from build123d import *

# Parameters (mm, degrees)
IZIM1_W               = 34
IZIM1_H               = 54
IZIM1_W_2             = 30
IZIM1_H_2             = 50
EKSTR_ZYON_NCE1_DEPTH = 50
KES_EKSTR_ZYON1_REACH = 81.75
IZIM2_R               = 4
IZIM2_R_2             = 2
EKSTR_ZYON_NCE2_DEPTH = 27


with BuildPart() as part:
    # Çizim1 → Ekstrüzyon-İnce1 (new body)
    with BuildSketch(Plane.XY):
        with Locations((15, 25)):
            Rectangle(IZIM1_W, IZIM1_H)
        with Locations((15, 25)):
            Rectangle(IZIM1_W_2, IZIM1_H_2, mode=Mode.SUBTRACT)
    extrude(amount=EKSTR_ZYON_NCE1_DEPTH)

    # Çizim2 → Kes-Ekstrüzyon1 (cut, up to next)
    with BuildSketch(Plane.ZY.offset(2), mode=Mode.PRIVATE) as kes_ekstr_zyon1_sk1:
        with Locations((25, 25)):
            Circle(IZIM2_R)
    kes_ekstr_zyon1_tool1 = extrude(kes_ekstr_zyon1_sk1.sketch, amount=-KES_EKSTR_ZYON1_REACH, mode=Mode.PRIVATE) & part.part
    # Çizim2 → Kes-Ekstrüzyon1 (cut, up to next)
    with BuildSketch(Plane.ZY.offset(2), mode=Mode.PRIVATE) as kes_ekstr_zyon1_sk2:
        with Locations((33, 25)):
            Circle(IZIM2_R_2)
    kes_ekstr_zyon1_tool2 = extrude(kes_ekstr_zyon1_sk2.sketch, amount=-KES_EKSTR_ZYON1_REACH, mode=Mode.PRIVATE) & part.part
    # Çizim2 → Kes-Ekstrüzyon1 (cut, up to next)
    with BuildSketch(Plane.ZY.offset(2), mode=Mode.PRIVATE) as kes_ekstr_zyon1_sk3:
        with Locations(Location((17, 25, 0), (0, 0, 180))):
            Circle(IZIM2_R_2)
    kes_ekstr_zyon1_tool3 = extrude(kes_ekstr_zyon1_sk3.sketch, amount=-KES_EKSTR_ZYON1_REACH, mode=Mode.PRIVATE) & part.part
    # Çizim2 → Kes-Ekstrüzyon1 (cut, up to next)
    with BuildSketch(Plane.ZY.offset(2), mode=Mode.PRIVATE) as kes_ekstr_zyon1_sk4:
        with Locations((25, 33)):
            Circle(IZIM2_R_2)
    kes_ekstr_zyon1_tool4 = extrude(kes_ekstr_zyon1_sk4.sketch, amount=-KES_EKSTR_ZYON1_REACH, mode=Mode.PRIVATE) & part.part
    # Çizim2 → Kes-Ekstrüzyon1 (cut, up to next)
    with BuildSketch(Plane.ZY.offset(2), mode=Mode.PRIVATE) as kes_ekstr_zyon1_sk5:
        with Locations(Location((25, 17, 0), (0, 0, 180))):
            Circle(IZIM2_R_2)
    kes_ekstr_zyon1_tool5 = extrude(kes_ekstr_zyon1_sk5.sketch, amount=-KES_EKSTR_ZYON1_REACH, mode=Mode.PRIVATE) & part.part
    add(kes_ekstr_zyon1_tool1.solids().sort_by_distance((-2, 25, 25))[0], mode=Mode.SUBTRACT)
    add(kes_ekstr_zyon1_tool2.solids().sort_by_distance((-2, 25, 33))[0], mode=Mode.SUBTRACT)
    add(kes_ekstr_zyon1_tool3.solids().sort_by_distance((-2, 25, 17))[0], mode=Mode.SUBTRACT)
    add(kes_ekstr_zyon1_tool4.solids().sort_by_distance((-2, 33, 25))[0], mode=Mode.SUBTRACT)
    add(kes_ekstr_zyon1_tool5.solids().sort_by_distance((-2, 17, 25))[0], mode=Mode.SUBTRACT)

    # Çizim3 → Ekstrüzyon-İnce2 (add, symmetric)
    with BuildSketch(Plane(origin=(0, 52, 0), x_dir=(1, 0, 0), z_dir=(0, 1, 0))):
        with BuildLine():
            ThreePointArc((25.118164338, -77.900907107), (30.254140884, -64.368544459), (32, -50))
            Line((32, -50), (32, 0))
            ThreePointArc((32, 0), (30.254140884, 14.368544459), (25.118164338, 27.900907107))
            Line((25.118164338, 27.900907107), (27.774072555, 29.295952462))
            ThreePointArc((27.774072555, 29.295952462), (33.166847928, 15.086971682), (35, 0))
            Line((35, 0), (35, -50))
            ThreePointArc((35, -50), (33.166847928, -65.086971682), (27.774072555, -79.295952462))
            Line((27.774072555, -79.295952462), (25.118164338, -77.900907107))
        make_face()
    ekstr_zyon_nce2 = extrude(amount=EKSTR_ZYON_NCE2_DEPTH, both=True)

    # Aynalama1: Ekstrüzyon-İnce2 across plane
    add(ekstr_zyon_nce2.mirror(Plane(origin=(-28, 25, 50), x_dir=(0, 0, 1), z_dir=(0, -1, 0))))


solid = part.part
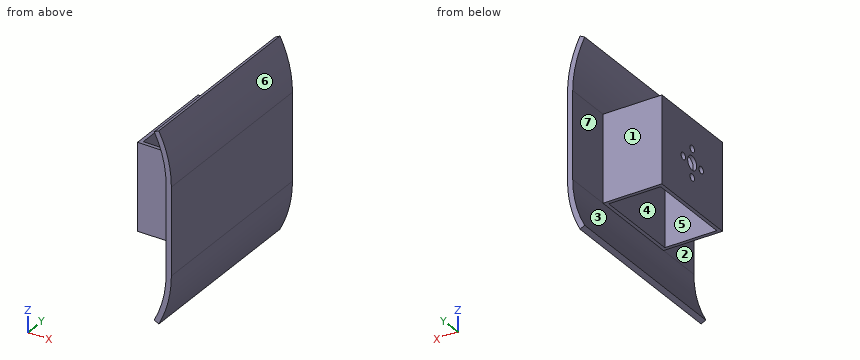
Here's how the part is built. I have some questions about the finished solid (model axes, mm). Face numbers are marked on the shaded views. A direction names the side the tool comes from. Coordinates: 2 decimals unless noted, no trailing zeros. Loops run counter-clockwise (first coordinate to the right, second up) from the corner with the lowest first, then second, coordinate; pieces in that order, holes last.
1. I need wall thicknesses on L1, parallel to X at y = 47, z = 38; L2, parallel to Y at x = 15.5, z = 16.5; L3, parallel to Z at x = -0.9, y = 17. Which ranges of each line are inside material? Lowest first, please.
2. Imagine slicing it at C-C, the plane z = 25. Please give me the cut outline in (x, y), and give its area (3 significant figures).
3. For P1, Ø10, axis at y = 58.5, z = -5.5, coming from the +X side; P2, Ø8, axis at y = 7, z = 64.5, coming from the -X side; P3, Ø2, axis at x = 26.5, y = 17.5, coming from the +Z side, each with a flat end and sliding along its axis, tell me the tip position at first contact or that it passes through.
4. For the marked faces 1, 2 and 3, which set-ups out of +Z, -Z, +X, -X, +Y, -Y let a thin tool reach every point of the face, with its end or its side?
5. Imagine slicing it at B-B, the plane x = 18. Please give me the cut outline in (y, z).
6. Imagine slicing it at A-A, the plane y = 33. Please give me the cut outline in (x, z), and give its area (3 significant figures).
7. If we mould it in two halves opening along X, with no side actions, what happens to the marked faces 4, 5, 6 and 7? For each: pulls with the +X half, pulls with the -X half, needs draft (parallel to the pull), parting line crosses it, or undercut.
8. Imagine slicing it at D-D, the plane y = 11.5. Please give me the cut outline in (x, z), and give its area (3 significant figures).
Taken from the geometry:
1. L1: x = -2 to 0, 30 to 35
1. L2: y = -2 to 0, 50 to 52
1. L3: z = 0 to 23, 27 to 50
2. outline: (-2, -2) - (32, -2) - (32, -29) - (35, -29) - (35, 79) - (32, 79) - (32, 52) - (-2, 52) - (-2, 35) - (0, 35) - (0, 50) - (30, 50) - (30, 0) - (0, 0) - (0, 15) - (-2, 15) - close; (-2, 19) - (0, 19) - (0, 21) - (-2, 21) - close; (-2, 29) - (0, 29) - (0, 31) - (-2, 31) - close
2. area: 628 mm2
3. P1: stops at x = 35
3. P2: stops at x = 29.08
3. P3: stops at z = 79.15
4. face 1: -X, +Y
4. face 2: -X, -Y
4. face 3: -X, +Y, -Y
5. outline: (-2, 0) - (0, 0) - (0, 50) - (-2, 50) - close; (50, 0) - (52, 0) - (52, 50) - (50, 50) - close
6. outline: (-2, 0) - (0, 0) - (0, 23) - (-2, 23) - close; (-2, 27) - (0, 27) - (0, 50) - (-2, 50) - close; (25.12, -27.9) - (27.77, -29.3) arc R63 ccw to (35, 0) - (35, 50) arc R63 ccw to (27.77, 79.3) - (25.12, 77.9) arc R60 cw to (32, 50) - (30, 50) - (30, 0) - (32, 0) arc R60 cw to start
6. area: 520 mm2
7. face 4: undercut
7. face 5: undercut
7. face 6: pulls with the +X half
7. face 7: pulls with the -X half
8. outline: (-2, 0) - (0, 0) - (0, 50) - (-2, 50) - close; (25.12, -27.9) - (27.77, -29.3) arc R63 ccw to (35, 0) - (35, 50) arc R63 ccw to (27.77, 79.3) - (25.12, 77.9) arc R60 cw to (32, 50) - (30, 50) - (30, 0) - (32, 0) arc R60 cw to start
8. area: 528 mm2
